```python
from build123d import *
from build123d.topology import SkipClean

# Parameters (mm, degrees)
BOSS_EXTRU_1_START      = 4.5
ESQUISSE1_R             = 2
BOSS_EXTRU_1_DEPTH      = 3
BOSS_EXTRU_2_START      = 7.5
BOSS_EXTRU_2_DEPTH      = 3.3
BOSS_EXTRU_5_START      = 8.3
ESQUISSE1_12_R          = 2
BOSS_EXTRU_5_DEPTH      = 2.5
BOSS_EXTRU_3_DEPTH      = 7.5
BOSS_EXTRU_4_START      = 0.5
BOSS_EXTRU_4_DEPTH      = 7
CONG_4_R                = 12
FILLET1_R               = 0.5
FILLET2_R               = 1
CHAMFER1_SIZE           = 2
ENL_V_START             = 4.5
ESQUISSE2_W             = 8
ESQUISSE2_H             = 18
ENL_V_MAT_EXTRU_1_DEPTH = 1
ENL_V_MAT_EXTRU_3_REACH = 52.206
ESQUISSE4_R             = 0.75
ESQUISSE5_W             = 21.366750419
ESQUISSE5_H             = 3.6
ENL_V_MAT_EXTRU_4_DEPTH = 1.1
CONG_5_R                = 1.1
ENL_V_MAT_EXTRU_5_REACH = 59.505
ESQUISSE12_R            = 0.75


# Some blends are built 0.0001 mm under size
with BuildPart() as part:
    # Esquisse1 → Boss.-Extru.1 (new body)
    with BuildSketch(Plane(origin=(0, 0, 0), x_dir=(0, 0, -1), z_dir=(1, 0, 0)).offset(BOSS_EXTRU_1_START)):
        with BuildLine():
            Line((30, 10), (0, 10))
            Line((0, 10), (0, 8))
            ThreePointArc((0, 8), (-8, 0), (0, -8))
            Line((0, -8), (30.291756081, -8))
            Line((30.291756081, -8), (30.291756081, 0))
            ThreePointArc((30.291756081, 0), (30.728647581, 2.879587526), (32, 5.5))
            Line((32, 5.5), (32, 8))
            Line((32, 8), (30, 10))
        make_face()
        Circle(ESQUISSE1_R, mode=Mode.SUBTRACT)
    extrude(amount=BOSS_EXTRU_1_DEPTH)

    # Esquisse1<8> → Boss.-Extru.2 (add)
    with BuildSketch(Plane(origin=(0, 0, 0), x_dir=(0, 0, -1), z_dir=(1, 0, 0)).offset(BOSS_EXTRU_2_START)):
        with BuildLine():
            Line((30, 10), (9.5, 10))
            Line((9.5, 10), (9.5, -8))
            Line((9.5, -8), (30.291756081, -8))
            Line((30.291756081, -8), (30.291756081, 0))
            ThreePointArc((30.291756081, 0), (30.728647581, 2.879587526), (32, 5.5))
            Line((32, 5.5), (32, 8))
            Line((32, 8), (30, 10))
        make_face()
    extrude(amount=BOSS_EXTRU_2_DEPTH)

    # Esquisse1<12> → Boss.-Extru.5 (add)
    with BuildSketch(Plane(origin=(0, 0, 0), x_dir=(0, 0, -1), z_dir=(1, 0, 0)).offset(BOSS_EXTRU_5_START)):
        with BuildLine():
            Line((40, 8), (32, 8))
            Line((32, 8), (32, 7))
            Line((32, 7), (32, 5.5))
            ThreePointArc((32, 5.5), (30.728647581, 2.879587526), (30.291756081, 0))
            Line((30.291756081, 0), (30.291756081, -8))
            Line((30.291756081, -8), (40, -8))
            ThreePointArc((40, -8), (48, 0), (40, 8))
        make_face()
        with Locations((40, 0)):
            Circle(ESQUISSE1_12_R, mode=Mode.SUBTRACT)
    extrude(amount=BOSS_EXTRU_5_DEPTH)

    # Esquisse1<9> → Boss.-Extru.3 (add)
    with BuildSketch(Plane(origin=(0, 0, 0), x_dir=(0, 0, -1), z_dir=(1, 0, 0))):
        with BuildLine():
            Line((0, 10), (2, 8))
            Line((2, 8), (28, 8))
            ThreePointArc((28, 8), (29.530733729, 8.30448187), (30.828427125, 9.171572875))
            Line((30.828427125, 9.171572875), (30, 10))
            Line((30, 10), (0, 10))
        make_face()
        with BuildLine():
            Line((0, 5.5), (28.791756081, 5.5))
            Line((28.791756081, 5.5), (28.791756081, -8))
            Line((28.791756081, -8), (30.291756081, -8))
            Line((30.291756081, -8), (30.291756081, 0))
            ThreePointArc((30.291756081, 0), (30.728647581, 2.879587526), (32, 5.5))
            Line((32, 5.5), (32, 7))
            Line((32, 7), (0, 7))
            ThreePointArc((0, 7), (-6.467156728, 2.678784027), (-4.949747468, -4.949747468))
            Line((-4.949747468, -4.949747468), (-3.889087297, -3.889087297))
            ThreePointArc((-3.889087297, -3.889087297), (-5.081337429, 2.104758878), (0, 5.5))
        make_face()
    extrude(amount=BOSS_EXTRU_3_DEPTH)

    # Esquisse1<10> → Boss.-Extru.4 (add)
    with BuildSketch(Plane(origin=(0, 0, 0), x_dir=(0, 0, -1), z_dir=(1, 0, 0)).offset(BOSS_EXTRU_4_START)):
        with BuildLine():
            Line((2, 8), (0, 10))
            Line((0, 10), (0, 8))
            ThreePointArc((0, 8), (-7.39103626, 3.061467459), (-5.656854249, -5.656854249))
            Line((-5.656854249, -5.656854249), (-4.949747468, -4.949747468))
            ThreePointArc((-4.949747468, -4.949747468), (-6.467156728, 2.678784027), (0, 7))
            Line((0, 7), (32, 7))
            Line((32, 7), (32, 8))
            Line((32, 8), (30.828427125, 9.171572875))
            ThreePointArc((30.828427125, 9.171572875), (29.530733729, 8.30448187), (28, 8))
            Line((28, 8), (2, 8))
        make_face()
    extrude(amount=BOSS_EXTRU_4_DEPTH)

    # Congé4
    # the kernel refuses this fillet: 12 mm, written as the material it takes off along each edge
    with BuildSketch(Plane(origin=(-11.583123952, 8, -2), x_dir=(0, 0, -1), z_dir=(1, 0, 0))) as cong_4_piece_1:
        with BuildLine():
            CenterArc((4.633249581, 12), CONG_4_R, 236.442690238, 33.557309762)
            Line((-2, 2), (-2.132664992, 1.8))
            ThreePointArc((-2.132664992, 1.8), (-1.169705627, 0.830294373), (-0.169705627, -0.169705627))
            Line((-0.169705627, -0.169705627), (0, -0.24))
            Line((0, -0.24), (4.633249581, -0.24))
            Line((4.633249581, -0.24), (4.633249581, 0))
        make_face()
    extrude(amount=12.083123952, mode=Mode.SUBTRACT)

    # Fillet1
    # the kernel refuses this fillet: 0.5 mm, written as the material it adds along each edge
    with BuildSketch(Plane(origin=(0.5, 20, -6.633249581), x_dir=(0, -0.7713363788823462, 0.6364276790120538), z_dir=(0, 0.6364276790120538, 0.7713363788823462))) as fillet1_piece_1_section:
        with BuildLine():
            CenterArc((12 + FILLET1_R, -FILLET1_R), FILLET1_R, 90, 90)
            Line((12 + FILLET1_R, 0), (12, 0))
            Line((12, 0), (12, -FILLET1_R))
        make_face()
    fillet1_piece_1 = revolve(axis=Axis((0.5, 20, -6.633249581), (1, 0, 0)), revolution_arc=39.525953359, mode=Mode.PRIVATE)
    fillet1_piece_1 = split(fillet1_piece_1, bisect_by=Plane(origin=(0.358961784, 10, -3.12843374), z_dir=(0, -1, 0)), keep=Keep.TOP, mode=Mode.PRIVATE)
    fillet1_piece_1 = split(fillet1_piece_1, bisect_by=Plane(origin=(0.358961784, 8.375840896, 0), z_dir=(0, 0, -1)), keep=Keep.TOP, mode=Mode.PRIVATE)
    add(fillet1_piece_1)
    with BuildSketch(Plane(origin=(0.5, 8, -28), x_dir=(-1, 0, 0), z_dir=(0, 0, 1))) as fillet1_piece_2:
        with BuildLine():
            CenterArc((FILLET1_R, FILLET1_R), FILLET1_R, 180, 90)
            Line((0, FILLET1_R), (0, 0))
            Line((0, 0), (FILLET1_R, 0))
        make_face()
    extrude(amount=21.366750419)
    with BuildSketch(Plane(origin=(0.5, 7, 0), x_dir=(-1, 0, 0), z_dir=(0, 0, -1))) as fillet1_piece_3:
        with BuildLine():
            CenterArc((FILLET1_R, FILLET1_R), FILLET1_R, 180, 90)
            Line((0, FILLET1_R), (0, 0))
            Line((0, 0), (FILLET1_R, 0))
        make_face()
    extrude(amount=32)
    with BuildSketch(Plane(origin=(0.5, 0, 0), x_dir=(0, -0.7071067811865441, 0.7071067811865509), z_dir=(0, -0.7071067811865509, -0.7071067811865441))) as fillet1_piece_4:
        with BuildLine():
            CenterArc((7 + FILLET1_R, FILLET1_R), FILLET1_R, 180, 90)
            Line((7 + FILLET1_R, 0), (7, 0))
            Line((7, 0), (7, FILLET1_R))
        make_face()
    revolve(axis=Axis((0.5, 0, 0), (-1, 0, 0)), revolution_arc=135)
    with BuildSketch(Plane(origin=(0.5, 12, -28), x_dir=(0, -0.7071067811865426, -0.7071067811865523), z_dir=(0, 0.7071067811865523, -0.7071067811865426))) as fillet1_piece_5:
        with BuildLine():
            CenterArc((4 + FILLET1_R, FILLET1_R), FILLET1_R, 180, 90)
            Line((4 + FILLET1_R, 0), (4, 0))
            Line((4, 0), (4, FILLET1_R))
        make_face()
    revolve(axis=Axis((0.5, 12, -28), (-1, 0, 0)), revolution_arc=45)

    # Fillet2
    fillet2_edges = [part.edges().sort_by_distance(p)[0] for p in [
        (4, 8, 0),
    ]]
    fillet(fillet2_edges, radius=FILLET2_R)

    # Chamfer1
    chamfer1_edges = [part.edges().sort_by_distance(p)[0] for p in [
        (10.8, 1, -9.5),
    ]]
    chamfer(chamfer1_edges, length=CHAMFER1_SIZE)

    # Symétrie1: part across plane


with BuildPart() as part_1:
    add(part.part)
    add(part.part.mirror(Plane(origin=(0, 0, 0), x_dir=(0, 0, 1), z_dir=(1, 0, 0))))

    # Esquisse2 → Enlèv. mat.-Extru.1 (cut)
    with SkipClean():  # the faces are left unmerged after this step: merging them gives an invalid solid
        with BuildSketch(Plane(origin=(0, 0, 0), x_dir=(0, 0, -1), z_dir=(1, 0, 0)).offset(ENL_V_START)):
            with Locations((-4, 1)):
                Rectangle(ESQUISSE2_W, ESQUISSE2_H)
        extrude(amount=-ENL_V_MAT_EXTRU_1_DEPTH, mode=Mode.SUBTRACT)

    # Esquisse4 → Enlèv. mat.-Extru.3 (cut, up to next)
    with BuildSketch(Plane.XY, mode=Mode.PRIVATE) as enl_v_mat_extru_3_sk1:
        with Locations((3.75, -3.8608)):
            Circle(ESQUISSE4_R)
    enl_v_mat_extru_3_tool1 = extrude(enl_v_mat_extru_3_sk1.sketch, amount=-ENL_V_MAT_EXTRU_3_REACH, mode=Mode.PRIVATE) & part_1.part
    add(enl_v_mat_extru_3_tool1.solids().sort_by_distance((3.75, -3.8608, 0))[0], mode=Mode.SUBTRACT)

    # Esquisse5 → Enlèv. mat.-Extru.4 (cut, symmetric)
    with SkipClean():  # the faces are left unmerged after this step: merging them gives an invalid solid
        with BuildSketch(Plane(origin=(0, 0, 0), x_dir=(0, 0, -1), z_dir=(1, 0, 0))):
            with Locations((17.316624791, 8.2)):
                Rectangle(ESQUISSE5_W, ESQUISSE5_H)
        extrude(amount=ENL_V_MAT_EXTRU_4_DEPTH, both=True, mode=Mode.SUBTRACT)

    # Congé5
    cong_5_edges = [part_1.edges().sort_by_distance(p)[0] for p in [
        (1.1, 6.4, -17.31662479),
        (-1.1, 6.4, -17.31662479),
    ]]
    fillet(cong_5_edges, radius=CONG_5_R - 0.0001)  # a hair under: the kernel refuses the full size

    # Esquisse10 → Enlèvement de matière-Révolution1 (revolve, cut)
    with BuildSketch(Plane.XY, mode=Mode.PRIVATE) as enl_vement_de_mati_re_r_volution1_sk:
        Polygon((-7.5, 5.15), (-6.9, 5.15), (-6.9, 4.5), (6.9, 4.5), (6.9, 5.15), (7.5, 5.15), (7.5, 2), (-7.5, 2), align=None)
    revolve(enl_vement_de_mati_re_r_volution1_sk.sketch.rotate(Axis((-7.5, 0, 0), (1, 0, 0)), 90), axis=Axis((-7.5, 0, 0), (1, 0, 0)), mode=Mode.SUBTRACT)

    # Esquisse12 → Enlèv. mat.-Extru.5 (cut, up to next)
    with BuildSketch(Plane(origin=(0, 7.263410428, 6.380108848), x_dir=(1, 0, 0), z_dir=(0, -0.7538821952908842, -0.6570096160813761)), mode=Mode.PRIVATE) as enl_v_mat_extru_5_sk1:
        with Locations(Location((-3.75, -4.165219968, 0), (0, 0, 136.743720403))):
            Circle(ESQUISSE12_R)
    enl_v_mat_extru_5_tool1 = extrude(enl_v_mat_extru_5_sk1.sketch, amount=ENL_V_MAT_EXTRU_5_REACH, mode=Mode.PRIVATE) & part_1.part
    add(enl_v_mat_extru_5_tool1.solids().sort_by_distance((-3.75, 10, 3.240024))[0], mode=Mode.SUBTRACT)


solid = part_1.part
```
Geometry check sheet. Reference: the model listing, model coordinates, mm. A direction names the side the tool comes from. Round coordinates to 2 decimals unless told otherwise and drop trailing zeros. Order: outer loops, then holes, each group sorted by start corner. A loop starts at its lowest first (then second) coordinate and runs counter-clockwise, first axis right, second up. Notation, with made-up numbers: M 41.5,84.5 L 97.5,84.5 A23 ccw 97.5,92.5 Z; hole C -6,27 d11. An arc over 180 degrees is marked long. Write item = value, one per line.
Q1. Scan lines: line 1 (X direction, y = -2.75, z = -38); line 2 (Y direction, x = -9.45, z = -40); line 3 (X direction, y = 2.5, z = -11.5). Record each from-to range of solid material in increasing order.
Answer block:
line_1 = -10.8 to -8.3, 8.3 to 10.8
line_2 = -8 to -2, 2 to 8
line_3 = -10.8 to -4.5, 4.5 to 10.8
Q2. Section check C-C (y = -6.25). Enter the section's corners in (x, z).
Answer block:
outline = M -10.8,-44.99 L -8.3,-44.99 L -8.3,-30.29 L 8.3,-30.29 L 8.3,-44.99 L 10.8,-44.99 L 10.8,-11.5 L 8.8,-9.5 L 7.5,-9.5 L 7.5,4.99 L 4.5,4.99 L 4.5,-28.79 L -4.5,-28.79 L -4.5,4.99 L -7.5,4.99 L -7.5,-9.5 L -8.8,-9.5 L -10.8,-11.5 Z
Q3. Set-up check for faces 1 (the cylindrical face through (7.2, 3.13, -4.09)), 2 (the flat face through (1.1, 9, -17)), 3 (the flat face through (4, 9, 0)), 4 (the flat face through (-3.8, 9.5, 0)): record each of +Z, -Z, +X, -X, +Y, -Y from which the full face is reachable in a straight line by a thin tool's end or side.
Answer block:
face_1 = +X
face_2 = +Y
face_3 = +Z, +Y
face_4 = +Z, +X, -X, +Y
Q4. Section check A-A (x = -1.75). Enter the section's corners in (y, z).
Answer block:
outline = M -8,-30.29 L 0,-30.29 A9.71 cw 5.5,-32 L 8,-32 L 10,-30 L 10,0 L 8.94,0 A1 cw 7.95,0.89 A8 ccw -5.66,5.66 L -3.89,3.89 A5.5 cw 5.5,0 L 5.5,-28.79 L -8,-28.79 Z
Q5. Release check for a two-part mould opening along Z. For faces 5 (the cylindrical face through (10, 0, -48)), 6 (the cylindrical face through (-5.68, -3.04, -3.32)), 7 (the cylindrical face through (-4.049, 8.285, 0.248)) record: released by +Z, released by -Z, zero draft, split by the parting line, or undercut.
Answer block:
face_5 = released by -Z
face_6 = undercut
face_7 = released by +Z
Q6. Depth check by flat-ended pin: pin 1 Ø1.3 at (x, y) = (-2, -2) entering from +Z; pin 2 Ø6 at (y, z) = (0, 0) entering from +X; pin 3 Ø6 at (x, y) = (-4, -1.5) entering from -Z; pin 4 Ø6.5 at (x, y) = (3, -3) entering from -Z (3 decimals). Enter the tip coordinate at first touch or a pass-through.
Answer block:
pin_1 = 7.89
pin_2 = through
pin_3 = -30.41
pin_4 = -30.295
